The drawing under review shows one solid part. Ordinate dimensions are in mm from its lowest x, y, z. A direction names the side the tool comes from. Give positions to 0.01 mm unless a question says otherwise; leave off trailing zeros. Loops run counter-clockwise (first coordinate to the right, second up) from the corner with the lowest first, then second, coordinate; pieces in that order, holes last. Notation, with made-up numbers: (71, 42) - (107, 42) arc R23 ccw to (107, 79) - close; hole circle Ø5 at (70, -25). An arc over 180 degrees is marked (long way). Write each question's results on one line, items separated by ' | '.
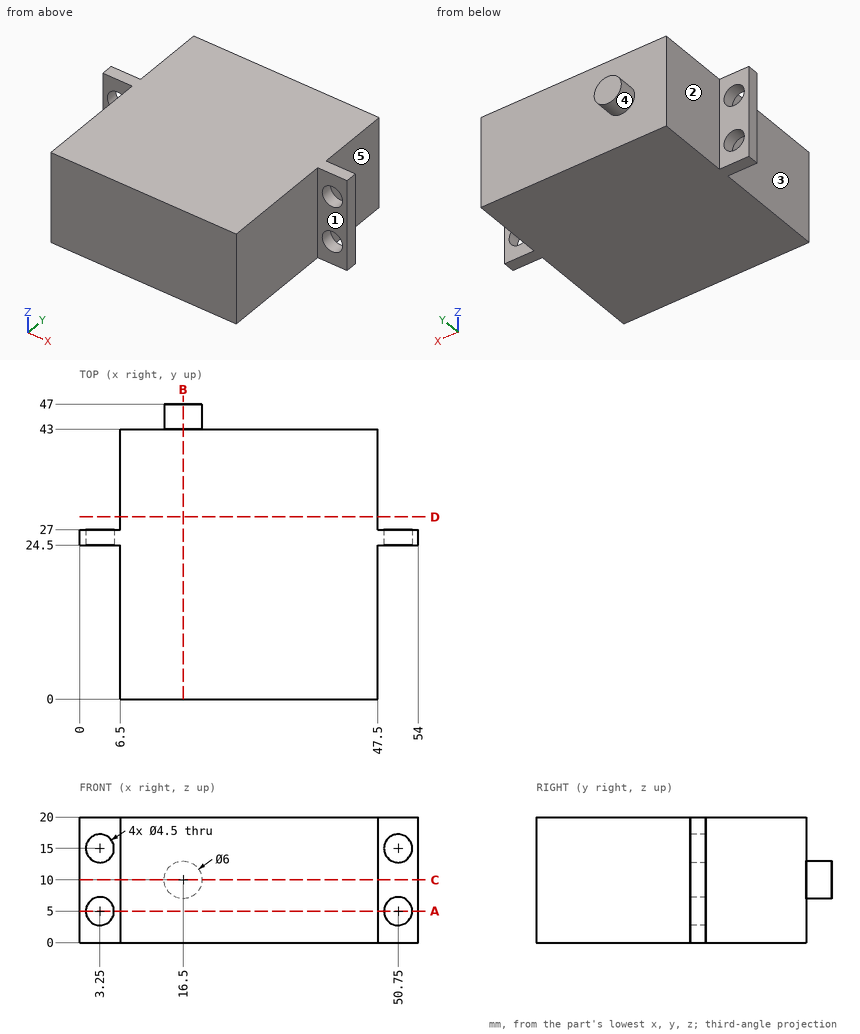
(1) Insertion check: P1, Ø10, axis at x = 42, z = 5.5, coming from the +Y side; P2, Ø10, axis at y = 10.5, z = 12.5, coming from the +X side; P3, Ø5, axis at x = 3.5, z = 9, coming from the +Y side; P4, Ø1, axis at x = 41.5, y = 41.5, coming from the -Z side. Each pin has a flat end and moves straight along its axis. Give the tip position at first contact, or say it passes through.
Answers below:
P1: y = 43 | P2: x = 47.5 | P3: y = 27 | P4: z = 0
(2) Wall thickness on line 1 along X through (y, z) = (25.1, 15); line 2 along Y through (x, z) = (34.5, 10.25); line 3 along X through (y, z) = (42, 8.5): over which ranges is each line inside the solid? List them lowest first. Write a range as from..to.
Answers below:
line 1: 0..1, 5.5..48.5, 53..54 | line 2: 0..43 | line 3: 6.5..47.5
(3) Take a section at B-B on x = 16.5. Give the boundary of the cut face in (y, z), plus the area to 3 significant figures.
Answers below:
outline: (0, 0) - (43, 0) - (43, 7) - (47, 7) - (47, 13) - (43, 13) - (43, 20) - (0, 20) - close | area: 884 mm2
(4) Take a section at A-A on z = 5. Give the boundary of the cut face in (x, y).
Answers below:
outline: (0, 24.5) - (1, 24.5) - (1, 27) - (0, 27) - close; (5.5, 24.5) - (6.5, 24.5) - (6.5, 0) - (47.5, 0) - (47.5, 24.5) - (48.5, 24.5) - (48.5, 27) - (47.5, 27) - (47.5, 43) - (6.5, 43) - (6.5, 27) - (5.5, 27) - close; (53, 24.5) - (54, 24.5) - (54, 27) - (53, 27) - close
(5) Take a section at D-D on y = 29. Give the boundary of the cut face in (x, z).
Answers below:
outline: (6.5, 0) - (47.5, 0) - (47.5, 20) - (6.5, 20) - close
(6) Take a section at C-C on z = 10. Give the boundary of the cut face in (x, y).
Answers below:
outline: (0, 24.5) - (6.5, 24.5) - (6.5, 0) - (47.5, 0) - (47.5, 24.5) - (54, 24.5) - (54, 27) - (47.5, 27) - (47.5, 43) - (19.5, 43) - (19.5, 47) - (13.5, 47) - (13.5, 43) - (6.5, 43) - (6.5, 27) - (0, 27) - close
(7) Tool access review of the marked faces 1, 2, 3, 4 and 5: name each direction out of +Z, -Z, +X, -X, +Y, -Y from which nothing blocks a thin tool from reaching the whole face with its end or side.
Answers below:
face 1: +Z, -Z, +X, -Y | face 2: +Z, -Z, -X, +Y | face 3: +Z, -Z, -X, -Y | face 4: +Y | face 5: +Z, -Z, +X, +Y
